For this review, take the finished solid that the model builds, in its own axes (mm). A direction names the side the tool comes from. Round coordinates to 2 decimals unless told otherwise and drop trailing zeros. Order: outer loops, then holes, each group sorted by start corner. A loop starts at its lowest first (then second) coordinate and runs counter-clockwise, first axis right, second up. Notation, with made-up numbers: (66.5, 1) -> (90.5, 1) arc R29 ccw to (90.5, 32) -> close; hole circle Ø6 at (87.25, 50). An arc over 180 degrees is marked (long way). Use a Markdown table: item, result. Add a question column.
1) Consider section A-A (x = 20.32). State the section outline as (y, z) points, plus the area to 3 significant figures.
2) Consider section C-C (y = 22.5). State the section outline as (x, z) points.
3) Clearance check with flat-ended pins moving along their axes: P1, Ø0.8, axis at y = 14, z = -56.5, coming from the -X side; P2, Ø2, axis at y = 15, z = -55, coming from the +X side; P3, Ø4, axis at x = 4.5, y = 24, coming from the +Z side. State where each tip first meets the part, or that it passes through.
4) Machinability: for faces 4 (the face through (103.886, 18, -57)), 5 (the face through (108, 18, -2.794)), 6 (the face through (110, 18, -53.086)), which of the approach directions +Z, -Z, +X, -X, +Y, -Y give a long, thin tool a straight path to every point of the face, cutting with its end or side? Answer none if there is none.
5) Draft analysis for pull direction Z (two halves, no side actions). For faces 1 (the face through (3.48, 17.96, -3.45)), 2 (the face through (17.84, 2.5, -44.47)), 3 (the face through (116.84, 3, -31)), state which applies: pulls with the +Z half, pulls with the -Z half, needs draft (parallel to the pull), parting line crosses it, or undercut.
6) Wall thickness on line 1 along Z through (x, y) = (7.5, 14.5); line 2 along X through (y, z) = (1.05, -17.78); line 3 along Z through (x, y) = (109, 10): over which ranges is each line inside the solid? List them lowest first. Write a range as [from, to].
7) Consider section D-D (z = -30.48). State the section outline as (x, y) points.
8) Consider section B-B (z = -17.78). State the section outline as (x, y) points, plus the area to 3 significant figures.
```python
from build123d import *

# Parameters (mm, degrees)
SKETCH1_W           = 111.76
SKETCH1_H           = 60.96
BOSS_EXTRUDE1_DEPTH = 5.08
FILLET1_R           = 5.08
CUT_EXTRUDE1_REACH  = 129.406
SKETCH3_R           = 2.794
SKETCH3_R_2         = 3.302
SKETCH5_W           = 10.16
SKETCH5_H           = 60.96
BOSS_EXTRUDE2_DEPTH = 5.08
FILLET2_R           = 5.08
SKETCH2_W           = 10.16
SKETCH2_H           = 10.16
SKETCH2_H_2         = 5.08
BOSS_EXTRUDE5_DEPTH = 25.4
FILLET9_R           = 2.286
FILLET10_R          = 5.08


with BuildPart() as part:
    # Sketch1 → Boss-Extrude1 (new body)
    with BuildSketch(Plane(origin=(0, 0, 0), x_dir=(1, 0, 0), z_dir=(0, 1, 0))):
        with Locations((55.88, 30.48)):
            Rectangle(SKETCH1_W, SKETCH1_H)
    extrude(amount=BOSS_EXTRUDE1_DEPTH)

    # Fillet1
    fillet1_edges = [part.edges().sort_by_distance(p)[0] for p in [
        (0, 2.54, -60.96),
        (111.76, 2.54, -60.96),
        (111.76, 2.54, 0),
        (0, 2.54, 0),
    ]]
    fillet(fillet1_edges, radius=FILLET1_R)

    # Sketch3 → Cut-Extrude1 (cut, up to next)
    with BuildSketch(Plane.XZ, mode=Mode.PRIVATE) as cut_extrude1_sk1:
        with Locations(Location((20.32, -17.78, 0), (0, 0, 270))):
            Circle(SKETCH3_R)
    cut_extrude1_tool1 = extrude(cut_extrude1_sk1.sketch, amount=-CUT_EXTRUDE1_REACH, mode=Mode.PRIVATE) & part.part
    # Sketch3 → Cut-Extrude1 (cut, up to next)
    with BuildSketch(Plane.XZ, mode=Mode.PRIVATE) as cut_extrude1_sk2:
        with Locations(Location((20.32, -43.18, 0), (0, 0, 270))):
            Circle(SKETCH3_R)
    cut_extrude1_tool2 = extrude(cut_extrude1_sk2.sketch, amount=-CUT_EXTRUDE1_REACH, mode=Mode.PRIVATE) & part.part
    # Sketch3 → Cut-Extrude1 (cut, up to next)
    with BuildSketch(Plane.XZ, mode=Mode.PRIVATE) as cut_extrude1_sk3:
        with Locations(Location((30.48, -30.48, 0), (0, 0, 270))):
            Circle(SKETCH3_R_2)
    cut_extrude1_tool3 = extrude(cut_extrude1_sk3.sketch, amount=-CUT_EXTRUDE1_REACH, mode=Mode.PRIVATE) & part.part
    add(cut_extrude1_tool1.solids().sort_by_distance((20.32, 0, -17.78))[0], mode=Mode.SUBTRACT)
    add(cut_extrude1_tool2.solids().sort_by_distance((20.32, 0, -43.18))[0], mode=Mode.SUBTRACT)
    add(cut_extrude1_tool3.solids().sort_by_distance((30.48, 0, -30.48))[0], mode=Mode.SUBTRACT)

    # Sketch5 → Boss-Extrude2 (add)
    with BuildSketch(Plane.XZ):
        with Locations((111.76, -30.48)):
            Rectangle(SKETCH5_W, SKETCH5_H)
    extrude(amount=-BOSS_EXTRUDE2_DEPTH)

    # Fillet2
    fillet2_edges = [part.edges().sort_by_distance(p)[0] for p in [
        (116.84, 2.54, 0),
        (116.84, 2.54, -60.96),
    ]]
    fillet(fillet2_edges, radius=FILLET2_R)

    # Sketch2 → Boss-Extrude5 (add)
    with BuildSketch(Plane(origin=(0, 5.08, 0), x_dir=(1, 0, 0), z_dir=(0, 1, 0))):
        with Locations((7.874, 53.086)):
            Rectangle(SKETCH2_W, SKETCH2_H)
        with Locations((7.874, 7.874)):
            Rectangle(SKETCH2_W, SKETCH2_H)
        with Locations((108.966, 55.626)):
            Rectangle(SKETCH2_W, SKETCH2_H_2)
        with Locations((108.966, 5.334)):
            Rectangle(SKETCH2_W, SKETCH2_H_2)
    extrude(amount=BOSS_EXTRUDE5_DEPTH)

    # Fillet9
    fillet9_edges = [part.edges().sort_by_distance(p)[0] for p in [
        (103.886, 17.78, -7.874),
        (114.046, 17.78, -2.794),
        (2.794, 17.78, -2.794),
        (2.794, 17.78, -58.166),
        (103.886, 17.78, -53.086),
        (114.046, 17.78, -58.166),
    ]]
    fillet(fillet9_edges, radius=FILLET9_R)

    # Fillet10
    fillet10_edges = [part.edges().sort_by_distance(p)[0] for p in [
        (12.954, 17.78, -12.954),
        (12.954, 17.78, -48.006),
    ]]
    fillet(fillet10_edges, radius=FILLET10_R)


solid = part.part
```
Results list:
| question | item | result |
|---|---|---|
| 1 | outline | (0, -60.96) -> (5.08, -60.96) -> (5.08, -45.97) -> (0, -45.97) -> close; (0, -40.39) -> (5.08, -40.39) -> (5.08, -20.57) -> (0, -20.57) -> close; (0, -14.99) -> (5.08, -14.99) -> (5.08, 0) -> (0, 0) -> close |
| 1 | area | 253 mm2 |
| 2 | outline | (2.79, -55.88) arc R2.29 ccw to (5.08, -58.17) -> (12.95, -58.17) -> (12.95, -53.09) arc R5.08 ccw to (7.87, -48.01) -> (2.79, -48.01) -> close; (2.79, -12.95) -> (7.87, -12.95) arc R5.08 ccw to (12.95, -7.87) -> (12.95, -2.79) -> (5.08, -2.79) arc R2.29 ccw to (2.79, -5.08) -> close; (103.89, -58.17) -> (111.76, -58.17) arc R2.29 ccw to (114.05, -55.88) -> (114.05, -53.09) -> (106.17, -53.09) arc R2.29 ccw to (103.89, -55.37) -> close; (103.89, -5.59) arc R2.29 ccw to (106.17, -7.87) -> (114.05, -7.87) -> (114.05, -5.08) arc R2.29 ccw to (111.76, -2.79) -> (103.89, -2.79) -> close |
| 3 | P1 | x = 2.8 |
| 3 | P2 | x = 114.05 |
| 3 | P3 | z = -2.79 |
| 4 | face 4 | +Z, -Z, +Y |
| 4 | face 5 | +Z, +X, -X, +Y |
| 4 | face 6 | +X, +Y |
| 5 | face 1 | pulls with the +Z half |
| 5 | face 2 | undercut |
| 5 | face 3 | needs draft |
| 6 | line 1 | [-58.17, -48.01], [-12.95, -2.79] |
| 6 | line 2 | [0, 17.53], [23.11, 116.84] |
| 6 | line 3 | [-58.17, -53.09], [-7.87, -2.79] |
| 7 | outline | (0, 0) -> (27.18, 0) -> (27.18, 5.08) -> (0, 5.08) -> close; (33.78, 0) -> (116.84, 0) -> (116.84, 5.08) -> (33.78, 5.08) -> close |
| 8 | outline | (0, 0) -> (17.53, 0) -> (17.53, 5.08) -> (0, 5.08) -> close; (23.11, 0) -> (116.84, 0) -> (116.84, 5.08) -> (23.11, 5.08) -> close |
| 8 | area | 565 mm2 |
